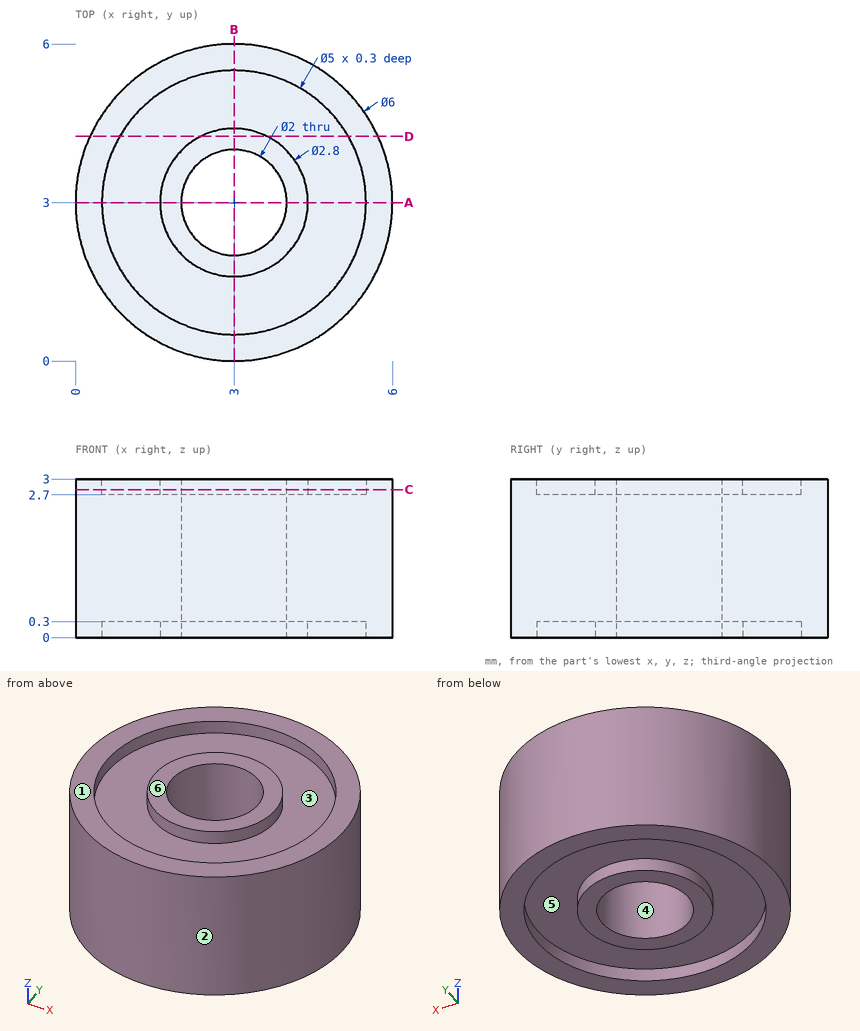
Job drawing, mm, ordinate dimensions from the low corner. One solid piece. A direction names the side the tool comes from. Give positions to 0.01 mm unless a question says otherwise; leave off trailing zeros. Loops run counter-clockwise (first coordinate to the right, second up) from the corner with the lowest first, then second, coordinate; pieces in that order, holes last. Notation, with made-up numbers: M 88,53 L 96,53 A20 ccw 96,80 Z; hole C 85,75 d6. An arc over 180 degrees is marked long. Use one line per item in the form item = value.
Item 1: Slice it at A-A on y = 3. List the corners of the cut face in (x, z).
Filled in:
outline = M 0,0 L 0.5,0 L 0.5,0.3 L 1.6,0.3 L 1.6,0 L 2,0 L 2,3 L 1.6,3 L 1.6,2.7 L 0.5,2.7 L 0.5,3 L 0,3 Z; M 4,0 L 4.4,0 L 4.4,0.3 L 5.5,0.3 L 5.5,0 L 6,0 L 6,3 L 5.5,3 L 5.5,2.7 L 4.4,2.7 L 4.4,3 L 4,3 Z
Item 2: Which spindle directions (+Z, -Z, +X, -X, +Y, -Y) get a long thin tool onto all of the face, cutting with end or side? Do the marked faces 5 and 6. Say none if no direction does.
Filled in:
face_5 = -Z
face_6 = +Z, +X, -X, +Y, -Y
Item 3: Two-plate mould, pull along Y, no slides. Class the marked faces 1, 2, 3 and 4: released by +Y, released by -Y, zero draft, split by the parting line, or undercut.
Filled in:
face_1 = zero draft
face_2 = split by the parting line
face_3 = undercut
face_4 = undercut
Item 4: Flat gauge pins, fed straight in: pin 1 Ø1.8 at (x, y) = (3, 3) entering from -Z (1 decimal); pin 2 Ø1 at (x, z) = (4.5, 1.5) entering from -Y. Where does each tip first touch, or does it go through?
Filled in:
pin_1 = through
pin_2 = 0.17
Item 5: Slice it at D-D on y = 4.25. List the corners of the cut face in (x, z).
Filled in:
outline = M 0.27,0 L 0.83,0 L 0.83,0.3 L 2.37,0.3 L 2.37,0 L 3.63,0 L 3.63,0.3 L 5.17,0.3 L 5.17,0 L 5.73,0 L 5.73,3 L 5.17,3 L 5.17,2.7 L 3.63,2.7 L 3.63,3 L 2.37,3 L 2.37,2.7 L 0.83,2.7 L 0.83,3 L 0.27,3 Z
Item 6: Slice it at C-C on z = 2.8. List the corners of the cut face in (x, y), and give its area (3 significant figures).
Filled in:
outline = C 3,3 d6; C 3,3 d2.8; hole C 3,3 d5; hole C 3,3 d2
area = 11.7 mm^2
Item 7: Drill centre lines: L1, parallel to Y at x = 3, z = 2.9; L2, parallel to Y at x = 3, z = 2.2; L3, parallel to Z at x = 0.9, y = 3.55. Where is each one in solid material? Low to high.
Filled in:
L1 = 0 to 0.5, 1.6 to 2, 4 to 4.4, 5.5 to 6
L2 = 0 to 2, 4 to 6
L3 = 0.3 to 2.7
